Work out the finished part from the listing and answer in its coordinate system (mm). Give positions to 0.01 mm unless a question says otherwise; leave off trailing zeros. Order: outer loops, then holes, each group sorted by start corner. A loop starts at its lowest first (then second) coordinate and runs counter-clockwise, first axis right, second up. Notation, with made-up numbers: M 22,18.5 L 58,18.5 A33 cw 58,49.5 Z; hole C 43.25,83.5 d8. An arc over 180 degrees is marked long. One line per item, written item: value.
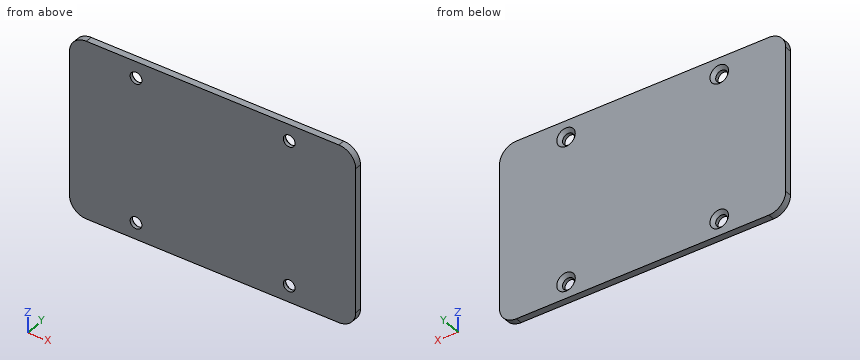
from build123d import *

# Parameters (mm, degrees)
SKETCH1_W           = 85
SKETCH1_H           = 52.8
BOSS_EXTRUDE1_DEPTH = 1
SKETCH2_R           = 1.75
CUT_EXTRUDE1_DEPTH  = 2
CHAMFER1_SIZE       = 1
FILLET2_R           = 5


with BuildPart() as part:
    # Sketch1 → Boss-Extrude1 (new, symmetric)
    with BuildSketch(Plane(origin=(0, 0, 0), x_dir=(1, 0, 0), z_dir=(0, 1, 0))):
        Rectangle(SKETCH1_W, SKETCH1_H)
    extrude(amount=BOSS_EXTRUDE1_DEPTH, both=True)

    # Sketch2 → Cut-Extrude1 (cut)
    with BuildSketch(Plane(origin=(0, 1, 0), x_dir=(1, 0, 0), z_dir=(0, 1, 0))):
        with Locations(Location((-22.75, 21.5, 0), (0, 0, 270))):
            Circle(SKETCH2_R)
        with Locations(Location((22.75, 21.5, 0), (0, 0, 270))):
            Circle(SKETCH2_R)
        with Locations(Location((22.75, -21.5, 0), (0, 0, 270))):
            Circle(SKETCH2_R)
        with Locations(Location((-22.75, -21.5, 0), (0, 0, 270))):
            Circle(SKETCH2_R)
    extrude(amount=-CUT_EXTRUDE1_DEPTH, mode=Mode.SUBTRACT)

    # Chamfer1
    chamfer1_edges = [part.edges().sort_by_distance(p)[0] for p in [
        (-22.75, 1, 19.75),
        (22.75, 1, 19.75),
        (22.75, 1, -23.25),
        (-22.75, 1, -23.25),
    ]]
    chamfer(chamfer1_edges, length=CHAMFER1_SIZE)

    # Fillet2
    fillet2_edges = [part.edges().sort_by_distance(p)[0] for p in [
        (42.5, 0, 26.4),
        (-42.5, 0, 26.4),
        (-42.5, 0, -26.4),
        (42.5, 0, -26.4),
    ]]
    fillet(fillet2_edges, radius=FILLET2_R)


solid = part.part
(1) Given P1, Ø4.5, axis at x = -22.75, z = 21.5, coming from the +Y side; P2, Ø3, axis at x = -22.75, z = -21.5, coming from the -Y side, each flat-ended and moving along its own axis, determine where each tip first touches the part or whether it passes through.
Findings:
P1: stops at y = 0.5
P2: passes through
(2) Section A-A, the plane x = -22.75 is taken. Give the vertices of the cut face in (y, z).
Findings:
outline: M -1,-26.4 L 1,-26.4 L 1,-24.25 L 0,-23.25 L -1,-23.25 Z; M -1,-19.75 L 0,-19.75 L 1,-18.75 L 1,18.75 L 0,19.75 L -1,19.75 Z; M -1,23.25 L 0,23.25 L 1,24.25 L 1,26.4 L -1,26.4 Z
(3) Section B-B, the plane y = 0.6 is taken. Give the vertices of the cut face in (x, z), then the cut area to 3 significant figures.
Findings:
outline: M -42.5,-21.4 A5 ccw -37.5,-26.4 L 37.5,-26.4 A5 ccw 42.5,-21.4 L 42.5,21.4 A5 ccw 37.5,26.4 L -37.5,26.4 A5 ccw -42.5,21.4 Z; hole C -22.75,-21.5 d4.7; hole C -22.75,21.5 d4.7; hole C 22.75,-21.5 d4.7; hole C 22.75,21.5 d4.7
area: 4,400 mm^2
(4) Find the intervals of material crossed by probe 1 along X at (y, z) = (-0.75, -21.5); probe 2 along X at (y, z) = (0, -20); probe 3 along Y at (x, z) = (22, -24), in increasing order. Write a range as from..to.
Findings:
probe 1: x = -42.5..-24.5, -21..21, 24.5..42.5
probe 2: x = -42.5..-23.65, -21.85..21.85, 23.65..42.5
probe 3: y = -1..0.86
